Verification items for the finished model (mm, model axes). A direction names the side the tool comes from. Give positions to 0.01 mm unless a question says otherwise; leave off trailing zeros. Write each loop counter-clockwise with the first axis right and the second up, starting at its lowest first coordinate (ties: lowest second). Pieces come first, ordered by that corner, then holes.
from build123d import *

# Parameters (mm, degrees)
SKETCH_R        = 60
PAD_DEPTH       = 23
POCKET_DEPTH    = 20
SKETCH002_R     = 10
PAD001_DEPTH    = 50
SKETCH005_R     = 2.8
POCKET001_DEPTH = 50.001
SKETCH006_R     = 4.7
POCKET002_DEPTH = 6
FILLET_R        = 26
CHAMFER_SIZE    = 2
FILLET001_R     = 6
FILLET002_R     = 3


with BuildPart() as part:
    # Sketch → Pad (new body)
    with BuildSketch(Plane.XY):
        with BuildLine():
            ThreePointArc((-78.765475, -14), (61.318839, -51.38093), (0, 80))
            Line((-150, 80), (0, 80))
            Line((-150, 80), (-150, 23.233627))
            Line((-150, 23.233627), (-78.765475, -14))
        make_face()
        Circle(SKETCH_R, mode=Mode.SUBTRACT)
    extrude(amount=PAD_DEPTH)

    # Sketch001 (on Face6 of Pad) → Pocket (cut)
    with BuildSketch(Plane(origin=(0, 0, 0), x_dir=(1, 0, 0), z_dir=(0, 0, -1))):
        with BuildLine():
            Line((-178.35, 70), (0, 70))
            ThreePointArc((0, -70), (70, 0), (0, 70))
            Line((-178.35, -70), (0, -70))
            Line((-178.35, 70), (-178.35, -70))
        make_face()
    extrude(amount=-POCKET_DEPTH, mode=Mode.SUBTRACT)

    # Sketch002 (on Face6 of Pocket) → Pad001 (join)
    with BuildSketch(Plane.XY.offset(23)):
        with Locations((57.547184, 55.57267)):
            Circle(SKETCH002_R)
        with Locations((-27.510509, 79.89632)):
            Circle(SKETCH002_R)
    extrude(amount=-PAD001_DEPTH)

    # Sketch005 (on Face5 of Pad001) → Pocket001 (cut, through all)
    with BuildSketch(Plane.XY.offset(23)):
        with Locations((-27.510509, 79.89632)):
            Circle(SKETCH005_R)
        with Locations((57.547184, 55.57267)):
            Circle(SKETCH005_R)
    extrude(amount=-POCKET001_DEPTH, mode=Mode.SUBTRACT)

    # Sketch006 (on Face15 of Pocket001) → Pocket002 (cut)
    with BuildSketch(Plane.XY.offset(23)):
        with Locations((-27.510509, 79.89632)):
            Circle(SKETCH006_R)
        with Locations((57.547184, 55.57267)):
            Circle(SKETCH006_R)
    extrude(amount=-POCKET002_DEPTH, mode=Mode.SUBTRACT)

    # Fillet
    fillet_edges = [part.edges().sort_by_distance(p)[0] for p in [
        (-150, 23.233627, 21.5),
        (-78.765475, -14, 21.5),
    ]]
    fillet(fillet_edges, radius=FILLET_R)

    # Chamfer
    chamfer_edges = [part.edges().sort_by_distance(p)[0] for p in [
        (-60, 0, 23),
    ]]
    chamfer(chamfer_edges, length=CHAMFER_SIZE)

    # Fillet001
    fillet001_edges = [part.edges().sort_by_distance(p)[0] for p in [
        (-150, 80, 11.5),
    ]]
    fillet(fillet001_edges, radius=FILLET001_R)

    # Fillet002
    fillet002_edges = [part.edges().sort_by_distance(p)[0] for p in [
        (-38.729833, -70, 10),
    ]]
    fillet(fillet002_edges, radius=FILLET002_R)


solid = part.part
Item 1: Sectioned sample at D-D on x = -83. Record the cut outline in (y, z), then the cut area to 3 significant figures.
Answer key:
outline: (-13.03, 20) - (70, 20) - (70, 0) - (80, 0) - (80, 23) - (-13.03, 23) - close
area: 479 mm2
Item 2: Depth check by flat-ended pin: pin 1 (4.5 mm diameter, centred on x = 56, y = 56.5, fed in from +Z); pin 2 (14 mm diameter, centred on x = -12.5, z = 7.5, fed in from +Y); pin 3 (6 mm diameter, centred on x = -74, z = 9.5, fed in from -Y). Enter the tip coordinate at first touch or a pass-through.
Answer key:
pin 1: stops at z = 17
pin 2: stops at y = 85.88
pin 3: stops at y = 70
Item 3: Release check for a two-part mould opening along X. For faces 1 (the face through (55.3, 53.9, -4.7)), 2 (the face through (-12, -70, 10)), 3 (the face through (-25, 78, 17)), 4 (the face through (-81.1, -15.1, 21.5)) record: released by +X, released by -X, zero draft, split by the parting line, or undercut.
Answer key:
face 1: undercut
face 2: zero draft
face 3: undercut
face 4: released by -X
Item 4: Sectioned sample at B-B on z = -14. Record the cut outline in (x, y), then the cut area to 3 significant figures.
Answer key:
outline: circle Ø20 at (-27.51, 79.9); circle Ø20 at (57.55, 55.57); hole circle Ø5.6 at (-27.51, 79.9); hole circle Ø5.6 at (57.55, 55.57)
area: 579 mm2
Item 5: Sectioned sample at A-A on y = 0. Record the cut outline in (x, z).
Answer key:
outline: (-105.55, 20) - (-60, 20) - (-60, 21) - (-62, 23) - (-105.55, 23) - close; (60, 20) - (70, 20) - (70, 0) - (80, 0) - (80, 23) - (62, 23) - (60, 21) - close
Item 6: Set-up check for faces 5 (the face through (62.03, 56.98, 20.04)), 6 (the face through (62.923, 64.005, -7.206)), 7 (the face through (-90, 70, 10)), 8 (the face through (-92, 80, 11)): record each of +Z, -Z, +X, -X, +Y, -Y from which the full face is reachable in a straight line by a thin tool's end or side.
Answer key:
face 5: +Z
face 6: -Z
face 7: -Z, -X, -Y
face 8: +Z, -Z, -X, +Y
Item 7: Sectioned sample at C-C on z = 7.5. Record the cut outline in (x, y), then the cut area to 3 significant figures.
Answer key:
outline: (-150, 70) - (-28.95, 70) arc R10 ccw to (-26.07, 70) - (0, 70) arc R70 cw to (0, -70) - (-24.49, -70) arc R3 ccw to (-25.45, -75.84) arc R80 ccw to (64.03, 47.96) arc R10 ccw (long way) to (50.16, 62.32) arc R80 ccw to (0, 80) - (-17.51, 80) arc R10 ccw to (-37.51, 80) - (-144, 80) arc R6 ccw to (-150, 74) - close; hole circle Ø5.6 at (-27.51, 79.9); hole circle Ø5.6 at (57.55, 55.57)
area: 4,340 mm2
Item 8: Scan lines: line 1 along Y through (x, z) = (41, 10); line 2 along Z through (x, y) = (-126, 35); line 3 along X through (y, z) = (0, 20.75). Record each from-to range of solid material in increasing order.
Answer key:
line 1: y = -68.69 to -56.74, 56.74 to 68.69
line 2: z = 20 to 23
line 3: x = -105.55 to -60, 60 to 80
